The model under review builds one solid part; all positions refer to its coordinate system, in mm. Face numbers are marked on the shaded views. A direction names the side the tool comes from. Coordinates: 2 decimals unless noted, no trailing zeros. Write each loop counter-clockwise with the first axis right and the second up, starting at its lowest first coordinate (ties: lowest second). Pieces come first, ordered by that corner, then holes.
1) Mouldability with a two-part tool opening along X and no side actions: class the marked faces 1, 2 and 3 as released by +X, released by -X, zero draft, split by the parting line, or undercut.
2) Machinability: for the marked faces 4 and 5, which of the approach directions +Z, -Z, +X, -X, +Y, -Y give a long, thin tool a straight path to every point of the face, cutting with its end or side? Answer none if there is none.
3) For P1, Ø5.5, axis at y = -10, z = -2, coming from the +X side; P2, Ø8.5, axis at y = -9, z = 0, coming from the -X side; P3, Ø3, axis at y = -10.5, z = -4, coming from the -X side, all flat-tipped, find the tip position at first contact; note any pin that passes through.
4) Add section A-A, the plane y = 0. State the section outline as (x, z) points, then the cut area to 3 significant figures.
5) Add section B-B, the plane z = 5.25. State the section outline as (x, y) points, then the cut area to 3 significant figures.
6) Add section C-C, the plane z = 1.75. Give the number of separate pieces and of enclosed holes in the cut face, then the cut area to 3 significant figures.
7) For line 1 (Y direction, x = 1.5, z = -2.25); line 2 (Z direction, x = -5.25, y = -9); line 3 (Y direction, x = 1.7, z = 0), list the stretches that pass through material, from the lowest coordinate up.
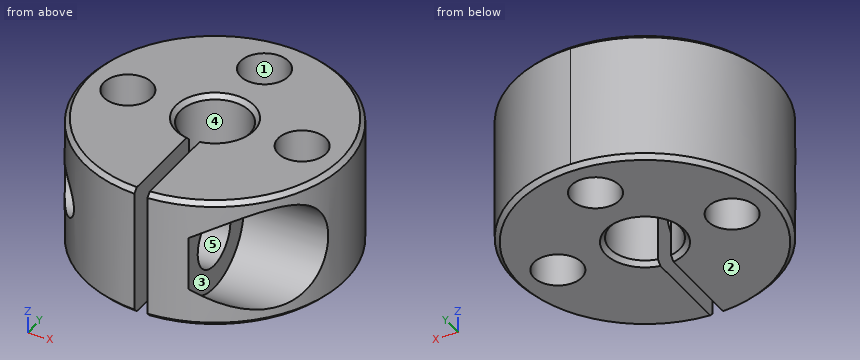
Autodesk Inventor part; units mm, degrees
ref_plane "to_bolt_XY" through (5, -9, 0) normal (1, 0, 0) x (0, 0, -1)
ref_plane "to_bolt_YZ" through (5, -9, 0) normal (0, 0, -1) x (0, 1, 0)
ref_plane "to_bolt_ZX" through (5, -9, 0) normal (0, 1, 0) x (1, 0, 0)
sketch "Sketch_14" plane through (0, 0, 0) normal (1, 0, 0) x (0, 1, 0)
  line L0 (0, -7.5) -> (0, 7.5)
  line L1 (0, 7.5) -> (14.5, 7.5)
  line L2 (14.5, 7.5) -> (15, 7)
  line L3 (15, 7) -> (15, -7)
  line L4 (15, -7) -> (14.5, -7.5)
  line L5 (14.5, -7.5) -> (0, -7.5)
  line L6 (0, -7.5) -> (0, 7.5)
revolve "Revolution1" add sketch "Sketch_14" angle 360 about axis through (0, 0, -7.5) along (0, 0, -1)
sketch "Sketch_15" plane through (0, 0, 0) normal (1, 0, 0) x (0, 1, 0)
  line L0 (0, -7.5) -> (0, 7.5)
  line L1 (0, 7.5) -> (4.5, 7.5)
  line L2 (4.5, 7.5) -> (4, 7)
  line L3 (4, 7) -> (4, -7)
  line L4 (4, -7) -> (4.5, -7.5)
  line L5 (4.5, -7.5) -> (0, -7.5)
  line L6 (0, -7.5) -> (0, 7.5)
revolve "Revolution2" cut sketch "Sketch_15" angle 360 about axis through (0, 0, -7.5) along (0, 0, -1)
sketch "Sketch_16" plane through (0, 0, 0) normal (0, 0, 1) x (1, 0, 0)
  arc A0 (-0.75, -15.9824) -> (0.75, -15.9824) centre (0, 0) ccw
  line L0 (0.75, -15.9824) -> (0.75, 0)
  line L1 (0.75, 0) -> (-0.75, 0)
  line L2 (-0.75, 0) -> (-0.75, -15.9824)
extrude "Extrusion1" cut sketch "Sketch_16" along normal mid plane 15
sketch "Sketch4" plane through (0, 0, -7.5) normal (0, 0, -1) x (-1, 0, 0)
  point P0 (-10, 0)
hole "Hole1" at (10, 0, -7.5) direction (0, 0, 1) diameter 5.5 depth 15
sketch "Sketch5" plane through (0, 0, -7.5) normal (0, 0, -1) x (-1, 0, 0)
  point P0 (10, 0)
hole "Hole2" at (-10, 0, -7.5) direction (0, 0, 1) diameter 5.5 depth 15
sketch "Sketch6" plane through (0, 0, -7.5) normal (0, 0, -1) x (-1, 0, 0)
  point P0 (0, 10)
hole "Hole3" at (0, 10, -7.5) direction (0, 0, 1) diameter 5.5 depth 15
sketch "Sketch_23" plane through (0, -9, 0) normal (0, 1, 0) x (1, 0, 0)
  line L0 (15, 0) -> (0, 0)
  line L1 (0, 0) -> (0, 3.3)
  line L2 (0, 3.3) -> (5, 3.3)
  line L3 (5, 3.3) -> (5, 6)
  line L4 (5, 6) -> (15, 6)
  line L5 (15, 6) -> (15, 0)
  line L6 (15, 0) -> (0, 0)
revolve "Revolution3" cut sketch "Sketch_23" angle 360 about axis through (15, -9, 0) along (1, 0, 0)
sketch "Sketch_25" plane through (0, 0, 0) normal (0, 0, 1) x (1, 0, 0)
  line L0 (-0.75, -9) -> (-13.7477, -9)
  line L1 (-13.7477, -9) -> (-13.7477, -6.5415)
  line L2 (-13.7477, -6.5415) -> (-1.2915, -6.5415)
  line L3 (-1.2915, -6.5415) -> (-0.75, -6)
  line L4 (-0.75, -6) -> (-0.75, -9)
  line L5 (-0.75, -9) -> (-13.7477, -9)
revolve "Revolution4" cut sketch "Sketch_25" angle 360 about axis through (-0.75, -9, 0) along (1, 0, 0)
thread "Thread1"
ref_plane "to_bolt_XY" through (5, -9, 0) normal (1, 0, 0) x (0, 0, -1)
ref_plane "to_bolt_YZ" through (5, -9, 0) normal (0, 0, -1) x (0, 1, 0)
ref_plane "to_bolt_ZX" through (5, -9, 0) normal (0, 1, 0) x (1, 0, 0)
properties part number "SCST8-15b"
Geometry results:
1. face 1: undercut
1. face 2: zero draft
1. face 3: released by +X
2. face 4: +Z, -Z
2. face 5: +X
3. P1: stops at x = 5
3. P2: stops at x = -14.23
3. P3: stops at x = -12
4. outline: (-15, -7) - (-14.5, -7.5) - (-12.75, -7.5) - (-12.75, 7.5) - (-14.5, 7.5) - (-15, 7) - close; (-7.25, -7.5) - (-4.5, -7.5) - (-4, -7) - (-4, 7) - (-4.5, 7.5) - (-7.25, 7.5) - close; (4, -7) - (4.5, -7.5) - (7.25, -7.5) - (7.25, 7.5) - (4.5, 7.5) - (4, 7) - close; (12.75, -7.5) - (14.5, -7.5) - (15, -7) - (15, 7) - (14.5, 7.5) - (12.75, 7.5) - close
4. area: 164 mm2
5. outline: (-0.75, -14.98) - (-0.75, -3.93) arc R4 cw (long way) to (0.75, -3.93) - (0.75, -14.98) arc R15 ccw to (9.13, -11.9) - (5, -11.9) - (5, -6.1) - (13.71, -6.1) arc R15 ccw (long way) to start; hole circle Ø5.5 at (-10, 0); hole circle Ø5.5 at (0, 10); hole circle Ø5.5 at (10, 0)
5. area: 529 mm2
6. separate pieces: 3
6. enclosed holes: 3
6. area: 435 mm2
7. line 1: y = -14.92 to -11.41, -6.59 to -3.71, 3.71 to 7.7, 12.3 to 14.92
7. line 2: z = -7.5 to -2.46, 2.46 to 7.5
7. line 3: y = -14.9 to -12.3, -5.7 to -3.62, 3.62 to 7.84, 12.16 to 14.9
